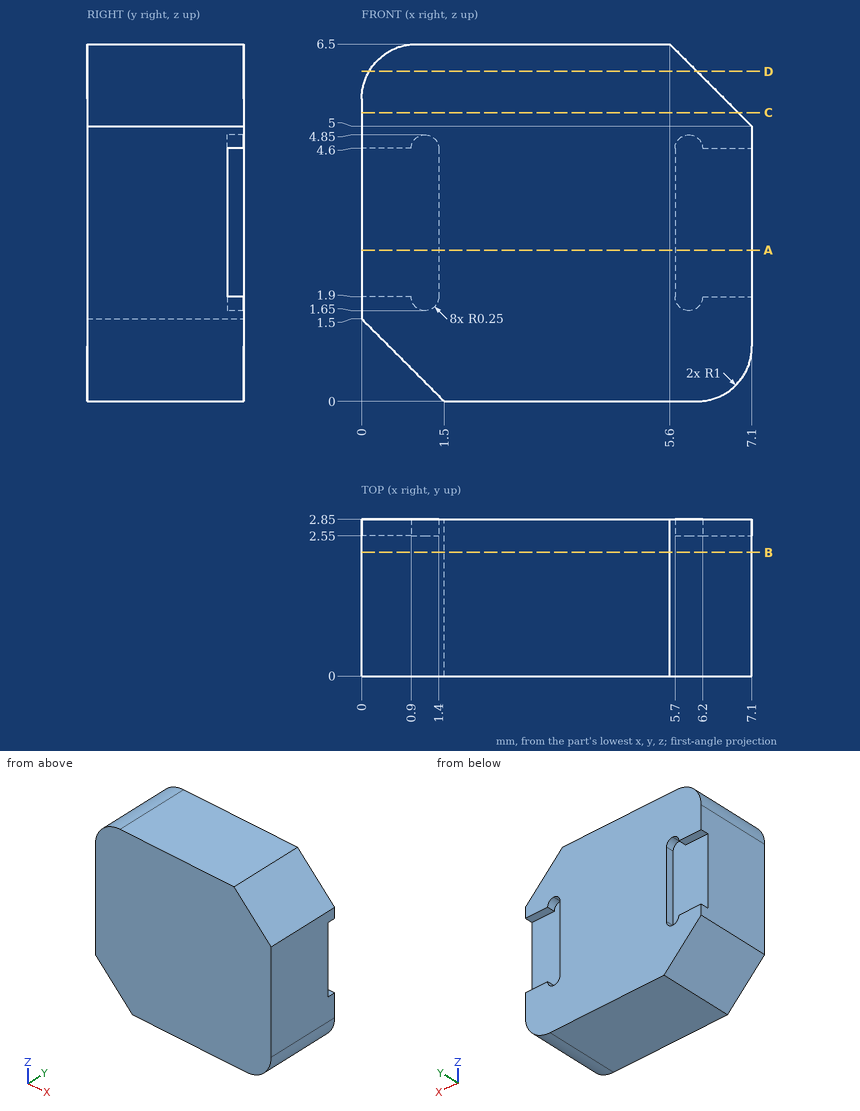
Study the drawing (mm; zero at the part's minimum x, y, z) and answer. Give positions to 0.01 mm unless a question says otherwise; leave off trailing zeros. Write each loop counter-clockwise with the first axis right and the second up, starting at its lowest first coordinate (ties: lowest second). Pieces come first, ordered by that corner, then holes. Notation, with made-up numbers: (62.25, -5.75) -> (110.25, -5.75) arc R30 cw to (110.25, 32.25) -> close; hole circle Ø5 at (-6.5, 33.5). An arc over 180 degrees is marked (long way). Write item = value, one per line. Start each with the question number.
1) The part is cut by section A-A, the plane z = 2.75. Determine the outline of the cut face in (x, y), and give its area (3 significant figures).
2) Straight lines are drawn through the part: line 1 along Y through (x, z) = (5.75, 3); line 2 along X through (y, z) = (2.75, 2.25); line 3 along Z through (x, y) = (1.25, 0.6). For each, find the intervals that lie inside material, in ascending order.
3) The part is cut by section D-D, the plane z = 6. Determine the outline of the cut face in (x, y), and give its area (3 significant figures).
4) The part is cut by section B-B, the plane y = 2.25. Determine the outline of the cut face in (x, z), and give its area (3 significant figures).
5) The part is cut by section C-C, the plane z = 5.25. Determine the outline of the cut face in (x, y).
Solutions:
q1.outline = (0, 0) -> (7.1, 0) -> (7.1, 2.55) -> (5.7, 2.55) -> (5.7, 2.85) -> (1.4, 2.85) -> (1.4, 2.55) -> (0, 2.55) -> close
q1.area = 19.4 mm²
q2.line_1 = 0 to 2.55
q2.line_2 = 1.4 to 5.7
q2.line_3 = 0.25 to 6.5
q3.outline = (0.13, 0) -> (6.1, 0) -> (6.1, 2.85) -> (0.13, 2.85) -> close
q3.area = 17.0 mm²
q4.outline = (0, 1.5) -> (1.5, 0) -> (6.1, 0) arc R1 ccw to (7.1, 1) -> (7.1, 5) -> (5.6, 6.5) -> (1, 6.5) arc R1 ccw to (0, 5.5) -> close
q4.area = 43.5 mm²
q5.outline = (0, 0) -> (6.85, 0) -> (6.85, 2.85) -> (0, 2.85) -> close
